Could you check a few things on this model? Use its own coordinates, in mm. Face numbers are marked on the shaded views. Round coordinates to 2 decimals unless told otherwise and drop trailing zeros. Write each loop counter-clockwise with the first axis right and the second up, starting at its lowest first coordinate (ties: lowest second). Pieces come first, ordered by that corner, then holes. Notation, with made-up numbers: M 39.25,-30.5 L 81.25,-30.5 A28 ccw 81.25,-3.5 Z; hole C 32.25,79 d10. An arc over 180 degrees is marked long. One line per item, written item: value. Start each with the question number.
(1) If I drill on L1, parallel to Y at x = 13.25, z = 0; L2, parallel to X at y = -12.5, z = -21; L3, parallel to Y at x = 0.5, z = 0, over which ranges is the centre line in solid material (lowest first)?
(2) Thinking about a two-plate mould opening in X: for the marked faces 1, 2 and 3, which applies, released by +X, released by -X, zero draft, split by the parting line, or undercut?
(3) I'm going to push flat-ended pins straight in: pin 1 Ø3 at (y, z) = (13.5, -12) entering from +X; pin 2 Ø2 at (x, z) = (1.5, -13.5) entering from -Y; pin 3 Ø8.5 at (y, z) = (0, 0) entering from +X; pin 4 Ø1 at (x, y) = (0, -18) entering from +Z. Where does each tip first touch, or does it pass through?
(4) I want a section at A-A on x = 2.5. Please give me the cut outline in (y, z), and give its area (3 significant figures).
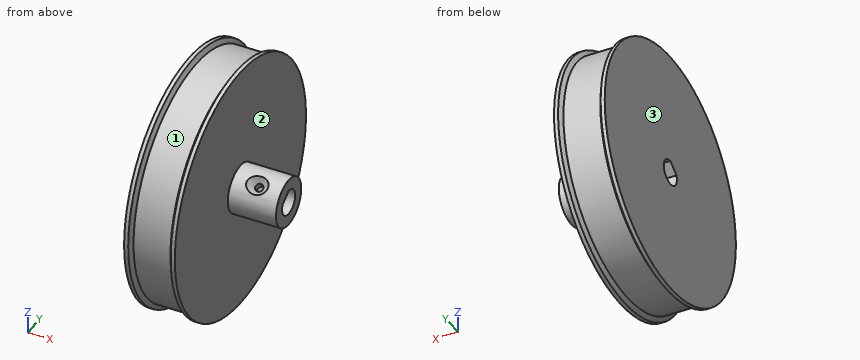
```python
from build123d import *

# Parameters (mm, degrees)
SKETCH1_R                                       = 25
BOSS_EXTRUDE1_DEPTH                             = 3.25
SKETCH2_R                                       = 26
BOSS_EXTRUDE2_DEPTH                             = 2
CUT_EXTRUDE1_DEPTH                              = 38.739236876
BOSS_EXTRUDE3_START                             = 10
SKETCH6_R                                       = 5
BOSS_EXTRUDE3_DEPTH                             = 10
CSK_FOR_M2_FLAT_HEAD_MACHINE_SCREW1_D           = 1.6
CSK_FOR_M2_FLAT_HEAD_MACHINE_SCREW1_DEPTH       = 5
CSK_FOR_M2_FLAT_HEAD_MACHINE_SCREW1_CSINK_D     = 4.4
CSK_FOR_M2_FLAT_HEAD_MACHINE_SCREW1_CSINK_ANGLE = 90
CSK_FOR_M2_FLAT_HEAD_MACHINE_SCREW1_TIP         = 0.480688495
CHAMFER3_SIZE                                   = 1.154700538
CHAMFER3_SIZE_2                                 = 2
CUT_EXTRUDE2_DEPTH                              = 10


# Read off the part's stored shape, not the designer's step: Mirror6
with BuildPart() as part:
    # Sketch1 → Boss-Extrude1 (new, symmetric)
    with BuildSketch(Plane(origin=(0, 0, 0), x_dir=(0, 0, -1), z_dir=(1, 0, 0))):
        Circle(SKETCH1_R)
    extrude(amount=BOSS_EXTRUDE1_DEPTH, both=True)

    # Sketch2 → Boss-Extrude2 (add)
    with BuildSketch(Plane(origin=(3.25, 0, 0), x_dir=(0, 0, -1), z_dir=(1, 0, 0))):
        Circle(SKETCH2_R)
    extrude(amount=BOSS_EXTRUDE2_DEPTH)

    # Sketch3 → Cut-Extrude1 (cut, symmetric)
    with BuildSketch(Plane(origin=(5.25, 0, 0), x_dir=(0, 0, -1), z_dir=(1, 0, 0))):
        with BuildLine():
            Line((-0.869230769, -2.450395452), (-2.6, 0))
            ThreePointArc((-2.6, 0), (2.123676058, 1.5), (-0.869230769, -2.450395452))
        make_face()
    extrude(amount=CUT_EXTRUDE1_DEPTH, both=True, mode=Mode.SUBTRACT)

    # Sketch6 → Boss-Extrude3 (add)
    with BuildSketch(Plane(origin=(5.25, 0, 0), x_dir=(0, 0, -1), z_dir=(1, 0, 0)).offset(BOSS_EXTRUDE3_START)):
        Circle(SKETCH6_R)
        with BuildLine():
            Line((-2.6, 0), (-0.869230769, -2.450395452))
            ThreePointArc((-0.869230769, -2.450395452), (2.123676058, 1.5), (-2.6, 0))
        make_face(mode=Mode.SUBTRACT)
    extrude(amount=-BOSS_EXTRUDE3_DEPTH)

    # CSK for M2 Flat Head Machine Screw1
    with Locations(Plane(origin=(0, -2.884615385, 4.08399242), x_dir=(0, -0.8167984839075115, -0.576923076923077), z_dir=(0, -0.576923076923077, 0.8167984839075115))):
        with Locations((0, 10.25)):
            CounterSinkHole(CSK_FOR_M2_FLAT_HEAD_MACHINE_SCREW1_D / 2, CSK_FOR_M2_FLAT_HEAD_MACHINE_SCREW1_CSINK_D / 2, depth=CSK_FOR_M2_FLAT_HEAD_MACHINE_SCREW1_DEPTH, counter_sink_angle=CSK_FOR_M2_FLAT_HEAD_MACHINE_SCREW1_CSINK_ANGLE)
            with Locations((0, 0, -(CSK_FOR_M2_FLAT_HEAD_MACHINE_SCREW1_DEPTH + CSK_FOR_M2_FLAT_HEAD_MACHINE_SCREW1_TIP / 2))):  # 118° drill point
                Cone(0, CSK_FOR_M2_FLAT_HEAD_MACHINE_SCREW1_D / 2, CSK_FOR_M2_FLAT_HEAD_MACHINE_SCREW1_TIP, mode=Mode.SUBTRACT)

    # Chamfer3
    # the kernel refuses this chamfer: 2, 1.154700538 mm, written as the material it takes off along each edge
    with BuildSketch(Plane(origin=(3.25, 0, 0), x_dir=(0, 0, -1), z_dir=(0, -1, 0))) as chamfer3_piece_1_section:
        Polygon((26, CHAMFER3_SIZE), (26 - CHAMFER3_SIZE_2, 0), (26, 0), align=None)
    chamfer3_piece_1 = revolve(axis=Axis((3.25, 0, 0), (1, 0, 0)), mode=Mode.PRIVATE)
    chamfer3_piece_1 = chamfer3_piece_1 - Plane(origin=(4.089516227, 0, 0), x_dir=(0, 0, -1), z_dir=(1, 0, 0)) * Cylinder(25, 105, mode=Mode.PRIVATE)
    add(chamfer3_piece_1, mode=Mode.SUBTRACT)

    # Mirror6 outline → Mirror6 (revolve)
    with BuildSketch(Plane.YX):
        Polygon((26, -5.25), (26, -4.404700538), (25, -3.827350269), (25, -3.25), (2.6, -3.25), (2.6, 3.25), (0, 3.25), (0, -5.25), align=None)
    revolve(axis=Axis((0, 0, 0), (1, 0, 0)))

    # Sketch12 → Cut-Extrude2 (cut)
    with BuildSketch(Plane(origin=(3.25, 0, 0), x_dir=(0, 0, -1), z_dir=(1, 0, 0))):
        with BuildLine():
            Line((-2.6, 0), (-0.869230769, -2.450395452))
            ThreePointArc((-0.869230769, -2.450395452), (2.123676058, 1.5), (-2.6, 0))
        make_face()
    extrude(amount=-CUT_EXTRUDE2_DEPTH, mode=Mode.SUBTRACT)


solid = part.part
```
Found:
1. L1: y = -5 to -2.6, 2.6 to 5
1. L2: x = -5.25 to 5.25
1. L3: y = -25 to -2.6, 2.6 to 25
2. face 1: undercut
2. face 2: released by +X
2. face 3: released by -X
3. pin 1: stops at x = 5.25
3. pin 2: stops at y = -21.65
3. pin 3: stops at x = 15.25
3. pin 4: stops at z = 17.85
4. outline: C 0,0 d50; hole M -2.45,0.87 A2.6 ccw long 0,2.6 Z
4. area: 1,940 mm²
